The model under review builds one solid part; all positions refer to its coordinate system, in mm. A direction names the side the tool comes from. Round coordinates to 2 decimals unless told otherwise and drop trailing zeros. Loops run counter-clockwise (first coordinate to the right, second up) from the corner with the lowest first, then second, coordinate; pieces in that order, holes last. Notation, with made-up numbers: (80.25, -21.75) -> (102.25, -21.75) arc R4 cw to (102.25, -16.75) -> close; hole circle Ø9 at (44.5, 1). An arc over 180 degrees is marked (long way). Return JSON: item names as keys, results as strings. Group by question number.
```python
from build123d import *

# Parameters (mm, degrees)
F0_W = 1.5
F0_H = 10
F2_R = 1.99999


# Not quite as in the source:
# - a fillet or chamfer is up to 0.001 mm smaller than in the source, because OpenCascade refuses the exact size


with BuildPart() as f1:
    # F0 (on Front) → F1 (revolve)
    with BuildSketch(Plane.XZ):
        with Locations((-0.75, 7)):
            Rectangle(F0_W, F0_H)
        Polygon((-15, 0), (0, 0), (0, 2), (-1.5, 2), (-15, 2), align=None)
    revolve(axis=Axis((0, 0, 27.7387052774), (0, 0, 1)))

    # F2 (radius 2 in the source; OpenCascade refuses exactly that, so slightly less here)
    f2_edges = [f1.edges().sort_by_distance(p)[0] for p in [
        (15, 0, 0),
        (1.5, 0, 2),
    ]]
    fillet(f2_edges, radius=F2_R)


solid = f1.part
```
1. We need section C-C, the plane z = 4.5. Write out the cut boundary in (x, y), then the cut area to 3 significant figures.
2. For P1, Ø2, axis at x = -8.5, y = -1.5, coming from the +Z side; P2, Ø2, axis at y = -2, z = 7, coming from the +X side; P3, Ø5, axis at y = 5, z = 6, coming from the -X side, all flat-tipped, find the tip position at first contact; note any pin that passes through.
3. Wall thickness on line 1 (Z direction, x = 10.75, y = -3.75); line 2 (Z direction, x = 13, y = 5); line 3 (X direction, y = -1.25, z = 10.5): over which ranges is each line inside the solid? List them lowest first.
4. Tool access review of faces 1 (the face through (0, 0, 0)), 2 (the face through (1.5, -0.07, 8.06)): name each direction out of +Z, -Z, +X, -X, +Y, -Y from which nothing blocks a thin tool from reaching the whole face with its end or side.
Check sheet entries:
{
 "1": {"outline": "circle Ø3 at (0, 0)", "area": "7.07 mm²"},
 "2": {"P1": "stops at z = 2", "P2": "stops at x = 1.12", "P3": "passes through"},
 "3": {"line 1": "z = 0 to 2", "line 2": "z = 0.23 to 2", "line 3": "x = -0.83 to 0.83"},
 "4": {"face 1": "-Z, +X, -X, +Y, -Y", "face 2": "+Z"}
}
